Answer from the drawing. Dimensions are ordinates in mm from the lowest x, y and z of the part. Round coordinates to 2 decimals unless told otherwise and drop trailing zeros. Write each loop counter-clockwise with the first axis right and the second up, starting at its lowest first coordinate (ties: lowest second). Pieces come first, ordered by that corner, then holes. Notation, with made-up numbers: (12, 39.25) - (57, 39.25) arc R20 ccw to (57, 72.25) - close; hole circle Ø1 at (9.25, -21). An arc over 180 degrees is marked (long way). Use a Markdown table: item, result. Add a question column.
1) A cutting plane is placed at B-B (x = 39). Give the vertices of the cut face in (y, z).
2) Each of these flat-tipped pins is pushed along its axis until it touches: P1, Ø2, axis at y = 2.5, z = 15, coming from the +X side; P2, Ø2, axis at x = 31.5, y = 5.5, coming from the -Z side; P3, Ø2, axis at y = 1.5, z = 14, coming from the -X side. Where does it stop, or does it pass through?
3) A cutting plane is placed at D-D (z = 70). Give the vertices of the cut face in (x, y).
4) Find the intervals of material crossed by probe 1 along Z at (x, y) = (30.5, 2.5) (3 decimals); probe 2 along Z at (x, y) = (24, 6.25); probe 3 along X at (y, z) = (2.25, 35), in increasing order. Write a range as from..to.
5) A cutting plane is placed at C-C (y = 1). Give the vertices of the cut face in (x, z).
6) A cutting plane is placed at A-A (x = 86). Give the vertices of the cut face in (y, z), then the cut area to 3 significant figures.
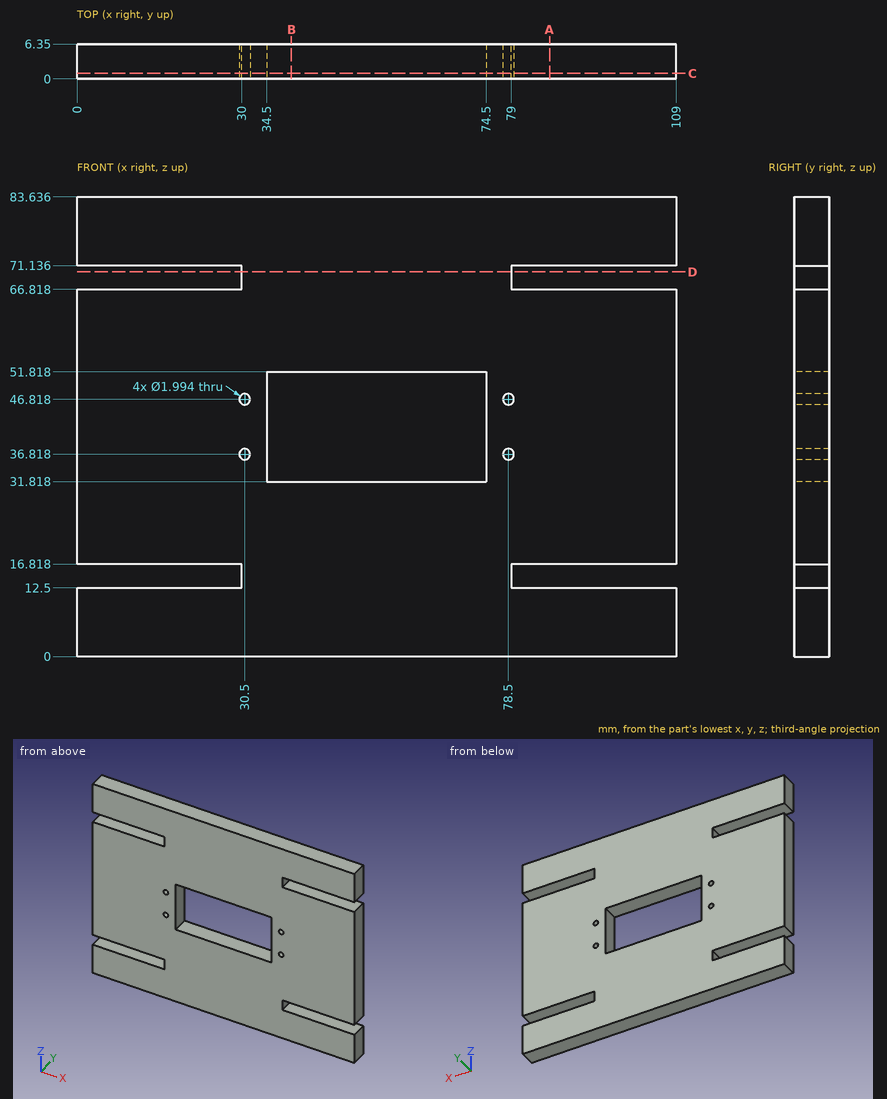
Entries:
| question | item | result |
|---|---|---|
| 1 | outline | (0, 0) - (6.35, 0) - (6.35, 31.82) - (0, 31.82) - close; (0, 51.82) - (6.35, 51.82) - (6.35, 83.64) - (0, 83.64) - close |
| 2 | P1 | stops at x = 79 |
| 2 | P2 | stops at z = 0 |
| 2 | P3 | stops at x = 30 |
| 3 | outline | (30, 0) - (79, 0) - (79, 6.35) - (30, 6.35) - close |
| 4 | probe 1 | z = 0..35.821, 37.815..45.821, 47.815..83.636 |
| 4 | probe 2 | z = 0..12.5, 16.82..66.82, 71.14..83.64 |
| 4 | probe 3 | x = 0..34.5, 74.5..109 |
| 5 | outline | (0, 0) - (109, 0) - (109, 12.5) - (79, 12.5) - (79, 16.82) - (109, 16.82) - (109, 66.82) - (79, 66.82) - (79, 71.14) - (109, 71.14) - (109, 83.64) - (0, 83.64) - (0, 71.14) - (30, 71.14) - (30, 66.82) - (0, 66.82) - (0, 16.82) - (30, 16.82) - (30, 12.5) - (0, 12.5) - close; hole circle Ø1.99 at (30.5, 36.82); hole circle Ø1.99 at (30.5, 46.82); hole (34.5, 31.82) - (74.5, 31.82) - (74.5, 51.82) - (34.5, 51.82) - close; hole circle Ø1.99 at (78.5, 36.82); hole circle Ø1.99 at (78.5, 46.82) |
| 6 | outline | (0, 0) - (6.35, 0) - (6.35, 12.5) - (0, 12.5) - close; (0, 16.82) - (6.35, 16.82) - (6.35, 66.82) - (0, 66.82) - close; (0, 71.14) - (6.35, 71.14) - (6.35, 83.64) - (0, 83.64) - close |
| 6 | area | 476 mm² |
